from build123d import *

# Parameters (mm, degrees)
BOSS_EXTRUDE1_DEPTH = 28.5
SKETCH2_R           = 1.35
CUT_EXTRUDE1_DEPTH  = 57
SKETCH3_W           = 8.922387131
SKETCH3_H           = 36.251387657
SKETCH3_R           = 1.65
SKETCH3_W_2         = 8
SKETCH3_H_2         = 60
BOSS_EXTRUDE2_DEPTH = 3


with BuildPart() as part:
    # Sketch1 → Boss-Extrude1 (new body, symmetric)
    with BuildSketch(Plane(origin=(0, 0, 0), x_dir=(0, 0, -1), z_dir=(1, 0, 0))):
        Polygon((-36.5, 0), (36.5, 0), (57.5, 10.700034439), (57.5, 13.700034439), (36.5, 3), (-36.5, 3), (-57.5, 13.700034439), (-57.5, 10.700034439), align=None)
    extrude(amount=BOSS_EXTRUDE1_DEPTH, both=True)

    # Sketch2 → Cut-Extrude1 (cut)
    with BuildSketch(Plane(origin=(0, 0, 0), x_dir=(1, 0, 0), z_dir=(0, 1, 0))):
        with Locations((-17.5, 17.5)):
            Circle(SKETCH2_R)
        with Locations((17.5, 17.5)):
            Circle(SKETCH2_R)
        with Locations((17.5, -17.5)):
            Circle(SKETCH2_R)
        with Locations((-17.5, -17.5)):
            Circle(SKETCH2_R)
        Polygon((-15, 20), (15, 20), (15, 15), (20, 15), (20, -15), (15, -15), (15, -20), (-15, -20), (-15, -15), (-20, -15), (-20, 15), (-15, 15), align=None)
    extrude(amount=CUT_EXTRUDE1_DEPTH, mode=Mode.SUBTRACT)

    # Sketch3 → Boss-Extrude2 (add)
    with BuildSketch(Plane(origin=(0, 0, 0), x_dir=(1, 0, 0), z_dir=(0, 1, 0))):
        with Locations((-32.961193565, 12.125693829)):
            Rectangle(SKETCH3_W, SKETCH3_H)
        with Locations((-32.5, 0)):
            Circle(SKETCH3_R, mode=Mode.SUBTRACT)
        with Locations((-32.5, 25.251387657)):
            Circle(SKETCH3_R, mode=Mode.SUBTRACT)
        with Locations((32.5, 0)):
            Rectangle(SKETCH3_W_2, SKETCH3_H_2)
        with Locations((32.5, -25)):
            Circle(SKETCH3_R, mode=Mode.SUBTRACT)
        with Locations((32.5, 25)):
            Circle(SKETCH3_R, mode=Mode.SUBTRACT)
    extrude(amount=BOSS_EXTRUDE2_DEPTH)


solid = part.part
Could you check a few things on this model? Use its own coordinates, in mm. A direction names the side the tool comes from. Give positions to 0.01 mm unless a question says otherwise; leave off trailing zeros. Write each loop counter-clockwise with the first axis right and the second up, starting at its lowest first coordinate (ties: lowest second). Pieces come first, ordered by that corner, then holes. Notation, with made-up numbers: (-12, 41) - (43, 41) arc R31 cw to (43, 65) - close; hole circle Ø6 at (-32, -12.75). An arc over 180 degrees is marked (long way). Use CSV: the item, a comma, the result in double quotes. Start each with the question number.
Item 1: I want a section at B-B, the plane x = 32.5. Please give me the cut outline in (y, z), then the cut area to 3 significant figures.
Item 2: For faces 1 (the face through (28.5, 5, -44)), 2 (the face through (32, 1, 30)), 3 (the face through (-18, 1, -15)), which set-ups out of +Z, -Z, +X, -X, +Y, -Y let a thin tool reach every point of the face, with its end or its side?
Item 3: I want a section at D-D, the plane x = 6. Please give me the cut outline in (y, z).
Item 4: I'm going to push flat-ended pins straight in: pin 1 (4 mm diameter, centred on x = 5, y = 8.5, fed in from -Z); pin 2 (2 mm diameter, centred on x = 32.5, z = 25, fed in from -Y); pin 3 (0.9 mm diameter, centred on x = -18, y = 2, fed in from +Z); pin 4 (6 mm diameter, centred on y = 9, z = -42.5, fed in from -X). Where does each tip first touch, or does it pass through?
Item 5: If we mould it in two halves opening along Z, with no side actions, what happens to faces 4 (the face through (16, 0, -16)), 5 (the face through (0.4, 8.3, 46.9)), 6 (the face through (32, 1, -30)), 7 (the face through (18.12, 1.48, -16.3))? For each: pulls with the +Z half, pulls with the -Z half, needs draft (parallel to the pull), parting line crosses it, or undercut.
Item 6: If I drill on line 1 along X through (y, z) = (2.25, -25); line 2 along X through (y, z) = (2.1, 0); line 3 along X through (y, z) = (2, -11), over which ranges is the centre line in solid material (lowest first)?
Item 7: I want a section at C-C, the plane x = -17.5. Please give me the cut outline in (y, z).
Item 8: I want a section at A-A, the plane z = 8.5. Please give me the cut outline in (x, y).
Findings:
1,outline,"(0, -30) - (3, -30) - (3, -26.65) - (0, -26.65) - close; (0, -23.35) - (3, -23.35) - (3, 23.35) - (0, 23.35) - close; (0, 26.65) - (3, 26.65) - (3, 30) - (0, 30) - close"
1,area,"160 mm2"
2,face 1,"-Z, +X, +Y, -Y"
2,face 2,"+Z, +X, +Y, -Y"
2,face 3,"+Y, -Y"
3,outline,"(0, -36.5) - (10.7, -57.5) - (13.7, -57.5) - (3, -36.5) - (3, -20) - (0, -20) - close; (0, 20) - (3, 20) - (3, 36.5) - (13.7, 57.5) - (10.7, 57.5) - (0, 36.5) - close"
4,pin 1,"stops at z = -57.11"
4,pin 2,"passes through"
4,pin 3,"stops at z = 41.31"
4,pin 4,"stops at x = -28.5"
5,face 4,"needs draft"
5,face 5,"undercut"
5,face 6,"pulls with the -Z half"
5,face 7,"undercut"
6,line 1,"x = -37.42 to -34.13, -30.87 to 30.85, 34.15 to 36.5"
6,line 2,"x = -37.42 to -34.15, -30.85 to -20, 20 to 36.5"
6,line 3,"x = -37.42 to -20, 20 to 36.5"
7,outline,"(0, -36.5) - (10.7, -57.5) - (13.7, -57.5) - (3, -36.5) - (3, -18.85) - (0, -18.85) - close; (0, -16.15) - (3, -16.15) - (3, -15) - (0, -15) - close; (0, 15) - (3, 15) - (3, 16.15) - (0, 16.15) - close; (0, 18.85) - (3, 18.85) - (3, 36.5) - (13.7, 57.5) - (10.7, 57.5) - (0, 36.5) - close"
8,outline,"(-28.5, 0) - (-20, 0) - (-20, 3) - (-28.5, 3) - close; (20, 0) - (36.5, 0) - (36.5, 3) - (20, 3) - close"
